For this review, take the finished solid that the model builds, in its own axes (mm). Face numbers are marked on the shaded views. Coordinates: 2 decimals unless noted, no trailing zeros. Order: outer loops, then holes, each group sorted by start corner. A loop starts at its lowest first (then second) coordinate and runs counter-clockwise, first axis right, second up. Notation, with made-up numbers: (-30, 69) -> (-2, 69) arc R8 cw to (-2, 74) -> close; hole circle Ø1 at (-5.75, -9). An arc over 180 degrees is marked (long way). Write item = value, one per line. Start each with the question number.
1) Wall thickness on probe 1 along X at (y, z) = (4, -7.5); probe 2 along Y at (x, z) = (2, -2.75); probe 3 along Y at (x, z) = (4.5, -6): over which ranges is each line inside the solid? List them lowest first. Write a range as [from, to].
2) Consider section D-D on x = 11.5. Give the boundary of the cut face in (y, z), and give its area (3 significant figures).
3) Draft analysis for pull direction X (two halves, no side actions). For the marked faces 1, 2 and 3, state which applies: +X half, -X half, draft (parallel to the pull), parting line (faces both ways), or undercut.
4) Consider section C-C on y = 137. Give the boundary of the cut face in (x, z), and give its area (3 significant figures).
5) Consider section A-A on z = -7. Give the boundary of the cut face in (x, y).
6) Insertion check: pin 1 Ø13 at (x, y) = (37.74, 137) entering from +Z. The pin has a flat end and moves straight along its axis. Give the tip position at first contact, or say it passes through.
7) Consider section B-B on y = 0. Give the boundary of the cut face in (x, z), and give its area (3 significant figures).
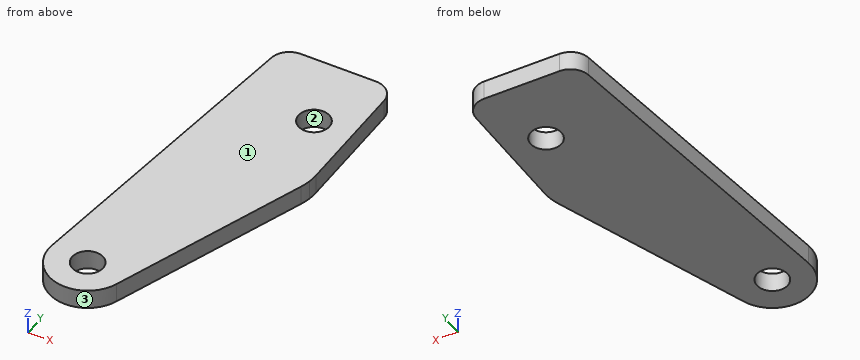
from build123d import *

# Parameters (mm, degrees)
SZKIC1_R                    = 20
SZKIC1_R_2                  = 8
DODANIE_WYCI_GNI_CIE1_DEPTH = 10


with BuildPart() as part:
    # Szkic1 → Dodanie-wyciągnięcie1 (new body)
    # profile 1 of 3: a face of its own
    with BuildSketch(Plane.XY):
        with BuildLine():
            Line((17.736087047, 99), (17.736087047, 175))
            Line((17.736087047, 175), (8.898572724, 175))
            ThreePointArc((8.898572724, 175), (2.243439653, 172.463859847), (-1.036023376, 166.141840763))
            Line((-1.036023376, 166.141840763), (-19.8691922, 2.283681526))
            ThreePointArc((-19.8691922, 2.283681526), (1.143712376, 19.967271271), (20, 0))
            ThreePointArc((20, 0), (19.69005749, -3.507368821), (18.769836395, -6.906029373))
            Line((18.769836395, -6.906029373), (55.890841639, 93.984823763))
            ThreePointArc((55.890841639, 93.984823763), (56.682391116, 96.462784094), (57.25630176, 99))
            Line((57.25630176, 99), (17.736087047, 99))
        make_face()
    # profile 2 of 3: a face of its own
    with BuildSketch(Plane.XY):
        Circle(SZKIC1_R)
        Circle(SZKIC1_R_2, mode=Mode.SUBTRACT)
    # profile 3 of 3: a face of its own
    with BuildSketch(Plane.XY):
        with BuildLine():
            Line((47.736087047, 175), (17.736087047, 175))
            Line((17.736087047, 175), (17.736087047, 99))
            Line((17.736087047, 99), (57.25630176, 99))
            ThreePointArc((57.25630176, 99), (57.615899976, 101.661186457), (57.736087047, 104.343867823))
            Line((57.736087047, 104.343867823), (57.736087047, 165))
            ThreePointArc((57.736087047, 165), (54.807154859, 172.071067812), (47.736087047, 175))
        make_face()
        with Locations((37.736087047, 137)):
            Circle(SZKIC1_R_2, mode=Mode.SUBTRACT)
    extrude(amount=-DODANIE_WYCI_GNI_CIE1_DEPTH)


solid = part.part
Answer sheet:
q1.probe_1 = [-19.67, -6.93], [6.93, 22.78]
q1.probe_2 = [-19.9, -7.75], [7.75, 172.24]
q1.probe_3 = [-19.49, -6.61], [6.61, 173.98]
q2.outline = (-16.36, -10) -> (175, -10) -> (175, 0) -> (-16.36, 0) -> close
q2.area = 1,910 mm2
q3.face_1 = draft
q3.face_2 = undercut
q3.face_3 = parting line
q4.outline = (-4.39, -10) -> (29.74, -10) -> (29.74, 0) -> (-4.39, 0) -> close; (45.74, -10) -> (57.74, -10) -> (57.74, 0) -> (45.74, 0) -> close
q4.area = 461 mm2
q5.outline = (-19.87, 2.28) arc R20 ccw to (18.77, -6.91) -> (55.89, 93.98) arc R30 ccw to (57.74, 104.34) -> (57.74, 165) arc R10 ccw to (47.74, 175) -> (8.9, 175) arc R10 ccw to (-1.04, 166.14) -> close; hole circle Ø16 at (0, 0); hole circle Ø16 at (37.74, 137)
q6.pin_1 = through
q7.outline = (-20, -10) -> (-8, -10) -> (-8, 0) -> (-20, 0) -> close; (8, -10) -> (21.31, -10) -> (21.31, 0) -> (8, 0) -> close
q7.area = 253 mm2
